Source: CAD feature listing. Evaluate the final solid. Frame: model axes, mm. A direction names the side the tool comes from. Round coordinates to 2 decimals unless told otherwise and drop trailing zeros. Order: outer loops, then holes, each group sorted by start corner. A loop starts at its lowest first (then second) coordinate and runs counter-clockwise, first axis right, second up. Notation, with made-up numbers: (56, 54.5) -> (65, 54.5) arc R13 cw to (65, 66.5) -> close; hole circle Ø11 at (19.5, 39). An arc over 180 degrees is marked (long way). One line per item, written item: value. Start each with the question number.
1) Section B-B (z = 0). Return the cut outline in (x, y).
2) Pin query (flat end, axial travel): P1, Ø1, axis at y = 2, z = -15.5, coming from the +X side. Return the tip coordinate at first contact, or that it passes through.
3) Section D-D (x = -21). Return the cut outline in (y, z).
4) Section C-C (y = 1.65). Return the cut outline in (x, z), and give its area (3 significant figures).
5) Mould query, pull axis Z, two halves, no side actions, for faces 1 (the face through (-29.775, 1.493, -6.612)), 2 (the face through (8, 0, -8)), 3 (the face through (9.76, 0.99, 31)). Classes: pulls with the +Z half, pulls with the -Z half, needs draft (parallel to the pull), parting line crosses it, or undercut.
6) Section A-A (x = 0). Return the cut outline in (y, z), and give its area (3 significant figures).
7) Reachability of faces 4 (the face through (4, 1, 10)), 5 (the face through (29, 2, -10)) from +Z, -Z, +X, -X, +Y, -Y: full face, straight path, thin tool, end or side. Return the list, or none.
8) Ray query, L1, parallel to X at y = 1.35, z = 0; L2, parallel to X at y = 1.4, z = 2; L3, parallel to X at y = 0.5, z = 0. Return the intervals inside material, ascending.
```python
from build123d import *

# Parameters (mm, degrees)
SZKIC1_R                    = 32.5
SZKIC1_R_2                  = 10.5
DODANIE_WYCI_GNI_CIE1_DEPTH = 1
SZKIC2_R                    = 32.5
SZKIC2_R_2                  = 30.5
SZKIC2_R_3                  = 24
SZKIC2_R_4                  = 22
SZKIC2_R_5                  = 16.5
SZKIC2_R_6                  = 14.5
DODANIE_WYCI_GNI_CIE2_DEPTH = 1


with BuildPart() as part:
    # Szkic1 → Dodanie-wyciągnięcie1 (new body)
    with BuildSketch(Plane(origin=(0, 0, 0), x_dir=(1, 0, 0), z_dir=(0, 1, 0))):
        with Locations(Location((0, 0, 0), (0, 0, 270))):
            Circle(SZKIC1_R)
        with Locations(Location((0, 0, 0), (0, 0, 270))):
            Circle(SZKIC1_R_2, mode=Mode.SUBTRACT)
    extrude(amount=DODANIE_WYCI_GNI_CIE1_DEPTH)

    # Szkic2 → Dodanie-wyciągnięcie2 (add)
    # profile 1 of 3: a face of its own
    with BuildSketch(Plane(origin=(0, 1, 0), x_dir=(1, 0, 0), z_dir=(0, 1, 0))):
        with Locations(Location((0, 0, 0), (0, 0, 270))):
            Circle(SZKIC2_R)
        with Locations(Location((0, 0, 0), (0, 0, 270))):
            Circle(SZKIC2_R_2, mode=Mode.SUBTRACT)
    # profile 2 of 3: a face of its own
    with BuildSketch(Plane(origin=(0, 1, 0), x_dir=(1, 0, 0), z_dir=(0, 1, 0))):
        with Locations(Location((0, 0, 0), (0, 0, 270))):
            Circle(SZKIC2_R_3)
        with Locations(Location((0, 0, 0), (0, 0, 270))):
            Circle(SZKIC2_R_4, mode=Mode.SUBTRACT)
    # profile 3 of 3: a face of its own
    with BuildSketch(Plane(origin=(0, 1, 0), x_dir=(1, 0, 0), z_dir=(0, 1, 0))):
        with Locations(Location((0, 0, 0), (0, 0, 270))):
            Circle(SZKIC2_R_5)
        with Locations(Location((0, 0, 0), (0, 0, 270))):
            Circle(SZKIC2_R_6, mode=Mode.SUBTRACT)
    extrude(amount=DODANIE_WYCI_GNI_CIE2_DEPTH)


solid = part.part
```
Findings:
1. outline: (-32.5, 0) -> (-10.5, 0) -> (-10.5, 1) -> (-14.5, 1) -> (-14.5, 2) -> (-16.5, 2) -> (-16.5, 1) -> (-22, 1) -> (-22, 2) -> (-24, 2) -> (-24, 1) -> (-30.5, 1) -> (-30.5, 2) -> (-32.5, 2) -> close; (10.5, 0) -> (32.5, 0) -> (32.5, 2) -> (30.5, 2) -> (30.5, 1) -> (24, 1) -> (24, 2) -> (22, 2) -> (22, 1) -> (16.5, 1) -> (16.5, 2) -> (14.5, 2) -> (14.5, 1) -> (10.5, 1) -> close
2. P1: x = 28.83
3. outline: (0, -24.8) -> (2, -24.8) -> (2, -22.12) -> (1, -22.12) -> (1, -11.62) -> (2, -11.62) -> (2, -6.56) -> (1, -6.56) -> (1, 6.56) -> (2, 6.56) -> (2, 11.62) -> (1, 11.62) -> (1, 22.12) -> (2, 22.12) -> (2, 24.8) -> (0, 24.8) -> close
4. outline: circle Ø65 at (0, 0); circle Ø48 at (0, 0); circle Ø33 at (0, 0); hole circle Ø61 at (0, 0); hole circle Ø44 at (0, 0); hole circle Ø29 at (0, 0)
4. area: 880 mm2
5. face 1: undercut
5. face 2: needs draft
5. face 3: parting line crosses it
6. outline: (0, -32.5) -> (2, -32.5) -> (2, -30.5) -> (1, -30.5) -> (1, -24) -> (2, -24) -> (2, -22) -> (1, -22) -> (1, -16.5) -> (2, -16.5) -> (2, -14.5) -> (1, -14.5) -> (1, -10.5) -> (0, -10.5) -> close; (0, 10.5) -> (1, 10.5) -> (1, 14.5) -> (2, 14.5) -> (2, 16.5) -> (1, 16.5) -> (1, 22) -> (2, 22) -> (2, 24) -> (1, 24) -> (1, 30.5) -> (2, 30.5) -> (2, 32.5) -> (0, 32.5) -> close
6. area: 56.0 mm2
7. face 4: +Y
7. face 5: +Z, -Z, +X, -X, +Y
8. L1: -32.5 to -30.5, -24 to -22, -16.5 to -14.5, 14.5 to 16.5, 22 to 24, 30.5 to 32.5
8. L2: -32.44 to -30.43, -23.92 to -21.91, -16.38 to -14.36, 14.36 to 16.38, 21.91 to 23.92, 30.43 to 32.44
8. L3: -32.5 to -10.5, 10.5 to 32.5
